```python
from build123d import *


with BuildPart() as part:
    # Sketch3 → Revolve1 (revolve)
    with BuildSketch(Plane(origin=(0, 0, 0), x_dir=(-1, 0, 0), z_dir=(0, 1, 0)), mode=Mode.PRIVATE) as revolve1_sk:
        with BuildLine():
            add(Edge.make_bspline(
                [(0, 7.5), (1.752854474, 5.664815439), (0.373820614, 7.240332376), (3.905572002, 2.879951334), (4.908772735, 4.915)],
                knots=[0, 0, 0, 0, 0.780983401, 1, 1, 1, 1], degree=3))
            Line((4.908772735, 4.915), (4.908772735, 0.915))
            Line((4.908772735, 0.915), (3.344098982, 0.778108784))
            ThreePointArc((3.344098982, 0.778108784), (3.040503625, 0.798007475), (2.756943239, 0.908278079))
            Line((2.756943239, 0.908278079), (0, 2.5))
            Line((0, 2.5), (-20, 2.5))
            Line((-20, 2.5), (-20, 5))
            Line((-20, 5), (-20, 7.5))
            Line((-20, 7.5), (0, 7.5))
        make_face()
        Polygon((-20, 10), (-20, 7.5), (-20, 5), (-34, 5), (-34, 10), align=None)
    revolve(revolve1_sk.sketch.rotate(Axis((0, 0, 0), (-1, 0, 0)), 180), axis=Axis((0, 0, 0), (-1, 0, 0)))


solid = part.part
```
Part model, mm, in its own coordinate system. A direction names the side the tool comes from. Round coordinates to 2 decimals unless told otherwise and drop trailing zeros. Order: outer loops, then holes, each group sorted by start corner. A loop starts at its lowest first (then second) coordinate and runs counter-clockwise, first axis right, second up. Notation, with made-up numbers: M 2,9.25 L 53,9.25 A8 ccw 53,14.25 Z; hole C 3,-37.5 d1. An arc over 180 degrees is marked long. Answer in a Markdown table with one row per item. Add a question column.
Q1. Cut at A-A on x = 13.5. Give the cut face in (y, z), and give its area (3 significant figures).
Q2. Wall check: L1, parallel to Y at x = 27.75, z = 0; L2, parallel to Y at x = 14.75, z = 0; L3, parallel to X at y = 0.5, z = -9. Give the ranges that are in metal, low to high. Write a range as from..to.
Q3. 3-axis set-ups, long thin cutter, end or side, ignore diameter. For faces 1 (the face through (27, 0, 5)), 2 (the face through (-4.909, -1.2, 0.1)), 3 (the face through (20, -7, -4)): which of +Z, -Z, +X, -X, +Y, -Y reach the whole face in a straight line?
Q4. Pin check, flat tips, straight feed: pin 1 (10 mm diameter, centred on x = 9, z = -2, fed in from +Y); pin 2 (1.5 mm diameter, centred on x = 10, z = -1.5, fed in from -Y); pin 3 (2 mm diameter, centred on x = 23.5, y = 6.5, fed in from +Z). Stop position of each tip, or through.
Q5. Cut at B-B on x = 22. Give the cut face in (y, z).
Q6. Mould opens along Z. For faces 4 (the face through (20, 2, 2)), 5 (the face through (34, -5, 2)), 6 (the face through (27, 0, 10)) say: +Z half, -Z half, draft (parallel to the pull), parting line (faces both ways), or undercut.
Established:
| question | item | result |
|---|---|---|
| 1 | outline | C 0,0 d15; hole C 0,0 d5 |
| 1 | area | 157 mm2 |
| 2 | L1 | y = -10..-5, 5..10 |
| 2 | L2 | y = -7.5..-2.5, 2.5..7.5 |
| 2 | L3 | x = 20..34 |
| 3 | face 1 | +X |
| 3 | face 2 | +Z, -Z, -X, +Y, -Y |
| 3 | face 3 | -X |
| 4 | pin 1 | stops at y = 7.5 |
| 4 | pin 2 | stops at y = -7.46 |
| 4 | pin 3 | stops at z = 8.35 |
| 5 | outline | C 0,0 d20; hole C 0,0 d10 |
| 6 | face 4 | undercut |
| 6 | face 5 | draft |
| 6 | face 6 | parting line |
